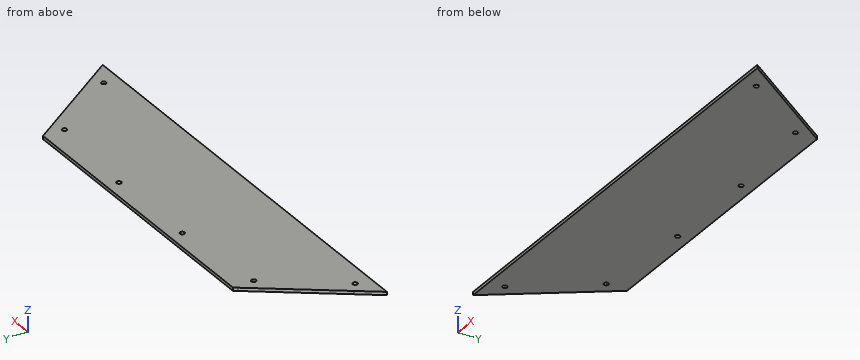
```python
from build123d import *

# Parameters (mm, degrees)
F0_R     = 2.3114
F1_DEPTH = 3.175


with BuildPart() as f1:
    # F0 (on Top) → F1 (new body)
    with BuildSketch(Plane.XY):
        with BuildLine():
            Line((-451.5609132883, 3.4527331373), (-420.9521720122, 3.4527331373))
            Line((-420.9521720122, 3.4527331373), (-359.0199119076, 91.1230753634))
            Line((-359.0199119076, 91.1230753634), (-379.4389155629, 105.5475091382))
            Line((-379.4389155629, 105.5475091382), (-386.6511324503, 95.3380073106))
            Line((-386.6511324503, 95.3380073106), (-378.3294900246, 89.4594158723))
            ThreePointArc((-378.3294900246, 89.4594158723), (-375.7419979554, 90.3287620732), (-374.1302306227, 88.1257904232))
            ThreePointArc((-374.1302306227, 88.1257904232), (-375.3786094336, 86.0733392273), (-377.7752560717, 86.2379310212))
            Line((-377.7752560717, 86.2379310212), (-424.151080008, 20.5890373971))
            ThreePointArc((-424.151080008, 20.5890373971), (-423.4322542612, 19.7641991843), (-423.1733054571, 18.7011779952))
            ThreePointArc((-423.1733054571, 18.7011779952), (-426.1843381244, 16.4982063451), (-427.3725648591, 20.0348034442))
            Line((-427.3725648591, 20.0348034442), (-435.6942072848, 25.9133948826))
            Line((-435.6942072848, 25.9133948826), (-451.5609132883, 3.4527331373))
        make_face()
        Polygon((-359.0199119076, 91.1230753634), (-420.9521720122, 3.4527331373), (-2.4390867117, 3.4527331373), (-77, 109), (-177, 109), (-227, 109), (-277, 109), (-377, 109), (-379.4389155629, 105.5475091382), align=None)
        with Locations((-28.5152945429, 18.7011779952)):
            Circle(F0_R, mode=Mode.SUBTRACT)
        with BuildLine():
            ThreePointArc((-274.6886, 96.5), (-278.634406614, 94.865593386), (-277, 98.8114))
            ThreePointArc((-277, 98.8114), (-275.365593386, 98.134406614), (-274.6886, 96.5))
        make_face(mode=Mode.SUBTRACT)
        with Locations((-77.5583693773, 88.1257904232)):
            Circle(F0_R, mode=Mode.SUBTRACT)
        with BuildLine():
            ThreePointArc((-174.6886, 96.5), (-177, 94.1886), (-179.3114, 96.5))
            ThreePointArc((-179.3114, 96.5), (-178.634406614, 98.134406614), (-177, 98.8114))
            ThreePointArc((-177, 98.8114), (-175.365593386, 98.134406614), (-174.6886, 96.5))
        make_face(mode=Mode.SUBTRACT)
        with BuildLine():
            Line((-415.5, 54.5), (-435.6942072848, 25.9133948826))
            Line((-435.6942072848, 25.9133948826), (-427.3725648591, 20.0348034442))
            ThreePointArc((-427.3725648591, 20.0348034442), (-425.8766080436, 20.9791117788), (-424.151080008, 20.5890373971))
            Line((-424.151080008, 20.5890373971), (-377.7752560717, 86.2379310212))
            ThreePointArc((-377.7752560717, 86.2379310212), (-378.7195644063, 87.7338878367), (-378.3294900246, 89.4594158723))
            Line((-378.3294900246, 89.4594158723), (-386.6511324503, 95.3380073106))
            Line((-386.6511324503, 95.3380073106), (-415.5, 54.5))
        make_face()
    extrude(amount=F1_DEPTH)


solid = f1.part
```
Check sheet for the modelled part. Datum: model origin and axes. Units: mm. Round coordinates to 2 decimals unless told otherwise and drop trailing zeros. Write each loop counter-clockwise with the first axis right and the second up, starting at its lowest first coordinate (ties: lowest second). Pieces come first, ordered by that corner, then holes. Notation, with made-up numbers: M 4.5,70.25 L 11.5,70.25 A14 ccw 11.5,82.25 Z; hole C 14,-24 d6. An arc over 180 degrees is marked long. Write item = value, one per line. Start each with the question number.
1. Scan lines: line 1 (X direction, y = 88, z = 1.5); line 2 (X direction, y = 87, z = 1.05); line 3 (Y direction, x = -277, z = 1.6). Record each from-to range of solid material in increasing order. Write a range as [from, to].
2. Section check A-A, the plane z = 1.55. Record the cut outline in (x, y).
3. Section check B-B, the plane x = -399. Record the cut outline in (y, z) (3 decimals), then the cut area to 3 significant figures.
4. Section check C-C, the plane y = 78.5. Record the cut outline in (x, z) (3 decimals), then the cut area to 3 significant figures.
Results found:
q1.line_1 = [-391.83, -378.75], [-374.13, -79.87], [-75.25, -62.17]
q1.line_2 = [-392.54, -378.46], [-374.42, -79.58], [-75.54, -61.46]
q1.line_3 = [3.45, 94.19], [98.81, 109]
q2.outline = M -451.56,3.45 L -2.44,3.45 L -77,109 L -377,109 Z; hole C -425.48,18.7 d4.62; hole C -376.44,88.13 d4.62; hole C -277,96.5 d4.62; hole C -177,96.5 d4.62; hole C -77.56,88.13 d4.62; hole C -28.52,18.7 d4.62
q3.outline = M 3.453,0 L 77.857,0 L 77.857,3.175 L 3.453,3.175 Z
q3.area = 236 mm^2
q4.outline = M -398.546,0 L -55.454,0 L -55.454,3.175 L -398.546,3.175 Z
q4.area = 1,090 mm^2
